For this review, take the finished solid that the model builds, in its own axes (mm). A direction names the side the tool comes from. Give positions to 0.01 mm unless a question says otherwise; leave off trailing zeros. Write each loop counter-clockwise with the first axis right and the second up, starting at its lowest first coordinate (ties: lowest second). Pieces come first, ordered by that corner, then holes. Notation, with made-up numbers: M 51,-8 L 109,-8 A26 ccw 109,24 Z; hole C 83.5,54.25 d2. An arc over 180 degrees is marked long. One line per item, written item: value. Start each with the question number.
Item 1: Consider section C-C, the plane y = -1.75. Write out the cut boundary in (x, z) (3 decimals), and give its area (3 significant figures).
Item 2: Consider section A-A, the plane z = 12.7. Write out the cut boundary in (x, y) (3 decimals).
Item 3: Consider section B-B, the plane y = 6.35. Write out the cut boundary in (x, z) (3 decimals), and give its area (3 significant figures).
Item 4: Tool access review of faces 1 (the face through (0, 3, 12)), 2 (the face through (-12, -6.35, 7)), 3 (the face through (-31.75, -0.2, 6.5)): name each direction out of +Z, -Z, +X, -X, +Y, -Y from which nothing blocks a thin tool from reaching the whole face with its end or side.
Item 5: Clearance check with flat-ended pins moving along their axes: pin 1 Ø3 at (x, y) = (-0.5, -10.5) entering from +Z; pin 2 Ø7.5 at (x, z) = (4, 10.5) entering from -Y; pin 3 Ø5 at (x, y) = (10, -4.5) entering from +Z; pin 4 Ø10 at (x, z) = (-22.098, 12.7) entering from -Y. State where each tip first meets the part, or that it passes through.
Item 6: To check wall thickness, follow probe 1 along Y at (x, z) = (-6.35, 13.75) (3 decimals); probe 2 along X at (y, z) = (-4.5, 12.7); probe 3 along Y at (x, z) = (-1, 1). State the ranges of each line that lie inside material, in increasing order.
Item 7: Consider section D-D, the plane z = 8. Write out the cut boundary in (x, y) (3 decimals), and give its area (3 significant figures).
Item 8: Mouldability with a two-part tool opening along Y and no side actions: class faces 4 (the face through (-4.6, 9, 12.8)), 5 (the face through (-7, -12.7, -9)), 6 (the face through (-7, 0, -3)), 7 (the face through (-16, 6, 6.35)) as released by +Y, released by -Y, zero draft, split by the parting line, or undercut.
```python
from build123d import *

# Parameters (mm, degrees)
F0_R     = 3.175
F1_DEPTH = 6.35
F3_DEPTH = 6.35
F4_W     = 31.75
F4_H     = 12.7
F4_R     = 3.175
F5_DEPTH = 12.7
F6_R     = 3.175
F7_DEPTH = 25.4


with BuildPart() as f1:
    # F0 (on Front) → F1 (new body)
    with BuildSketch(Plane.XZ):
        Polygon((19.05, 0), (0, 0), (0, 19.05), (-31.75, 19.05), (-31.75, -12.7), (19.05, -12.7), align=None)
        with Locations((-22.098, 12.7)):
            Circle(F0_R, mode=Mode.SUBTRACT)
    extrude(amount=F1_DEPTH)

    # F2 (on face) → F3 (join)
    with BuildSketch(Plane.XZ.offset(6.35)):
        Polygon((19.05, -6.35), (0, -6.35), (-31.75, -6.35), (-31.75, -12.7), (0, -12.7), (19.05, -12.7), align=None)
    extrude(amount=F3_DEPTH)

    # F4 (on face) → F5 (join)
    with BuildSketch(Plane(origin=(0, 0, 0), x_dir=(-1, 0, 0), z_dir=(0, 1, 0))):
        with Locations((15.875, 12.7)):
            Rectangle(F4_W, F4_H)
        with Locations((22.098, 12.7)):
            Circle(F4_R, mode=Mode.SUBTRACT)
    extrude(amount=F5_DEPTH)

    # F6 (on face) → F7 (cut)
    with BuildSketch(Plane.XY.offset(19.05)):
        with Locations((-6.35, 6.35)):
            Circle(F6_R)
    extrude(amount=-F7_DEPTH, mode=Mode.SUBTRACT)


solid = f1.part
```
Model answer:
1. outline: M -31.75,-12.7 L 19.05,-12.7 L 19.05,0 L 0,0 L 0,19.05 L -31.75,19.05 Z; hole C -22.098,12.7 d6.35
1. area: 1,220 mm2
2. outline: M -31.75,-6.35 L -25.273,-6.35 L -25.273,12.7 L -31.75,12.7 Z; M -18.923,-6.35 L 0,-6.35 L 0,12.7 L -18.923,12.7 Z; hole C -6.35,6.35 d6.35
3. outline: M -31.75,6.35 L -9.525,6.35 L -9.525,19.05 L -31.75,19.05 Z; M -3.175,6.35 L 0,6.35 L 0,19.05 L -3.175,19.05 Z; hole C -22.098,12.7 d6.35
3. area: 291 mm2
4. face 1: +Z, +X, +Y, -Y
4. face 2: +Z, +X, -X, -Y
4. face 3: +Z, -Z, -X, +Y, -Y
5. pin 1: stops at z = -6.35
5. pin 2: passes through
5. pin 3: stops at z = 0
5. pin 4: stops at y = -6.35
6. probe 1: y = -6.35 to 3.175, 9.525 to 12.7
6. probe 2: x = -31.75 to -25.27, -18.92 to 0
6. probe 3: y = -6.35 to 0
7. outline: M -31.75,-6.35 L 0,-6.35 L 0,12.7 L -31.75,12.7 Z; hole C -6.35,6.35 d6.35
7. area: 573 mm2
8. face 4: undercut
8. face 5: released by -Y
8. face 6: released by +Y
8. face 7: zero draft
